For this review, use the dimensioned drawing (mm, ordinates from the lowest corner) and the shaded views. Round coordinates to 2 decimals unless told otherwise and drop trailing zeros. Write each loop counter-clockwise with the first axis right and the second up, starting at its lowest first coordinate (ties: lowest second). Pieces come first, ordered by that corner, then holes. Notation, with made-up numbers: M 58.25,1.25 L 66.25,1.25 A22 cw 66.25,8.25 Z; hole C 83,64 d7. An arc over 180 degrees is marked long. One line per question, with ' | ' between items.
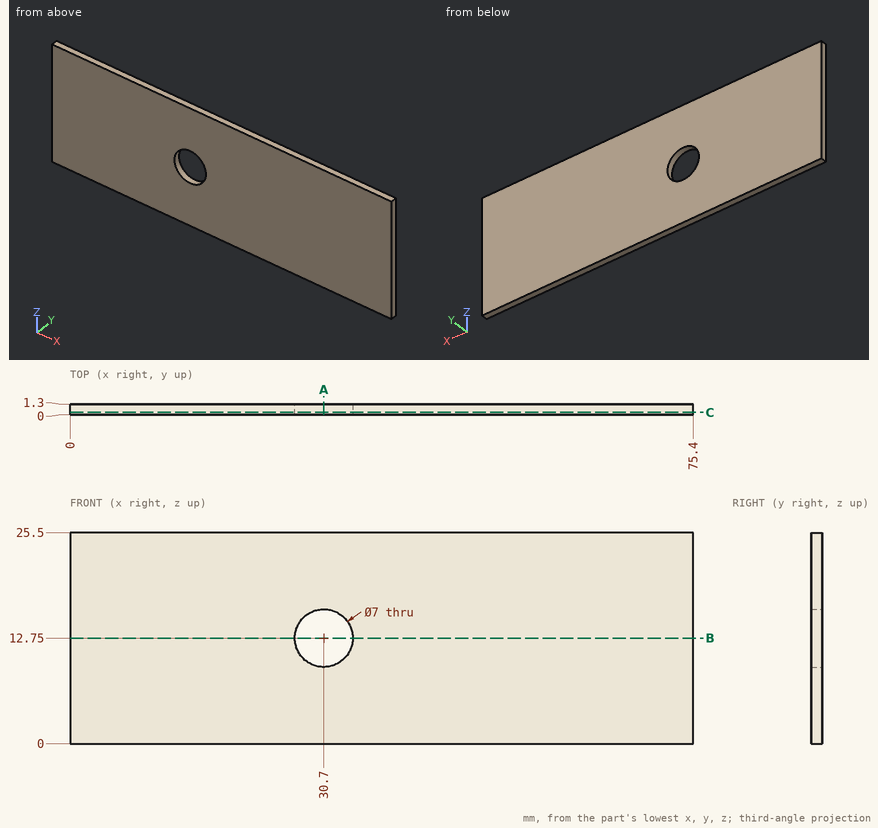
Item 1: Take a section at A-A (x = 30.7). Write out the cut boundary in (y, z).
Results:
outline: M 0,0 L 1.3,0 L 1.3,9.25 L 0,9.25 Z; M 0,16.25 L 1.3,16.25 L 1.3,25.5 L 0,25.5 Z
Item 2: Take a section at B-B (z = 12.75). Write out the cut boundary in (x, y).
Results:
outline: M 0,0 L 27.2,0 L 27.2,1.3 L 0,1.3 Z; M 34.2,0 L 75.4,0 L 75.4,1.3 L 34.2,1.3 Z
Item 3: Take a section at C-C (y = 0.3). Write out the cut boundary in (x, z).
Results:
outline: M 0,0 L 75.4,0 L 75.4,25.5 L 0,25.5 Z; hole C 30.7,12.75 d7
Item 4: To check wall thickness, follow line 1 along Z through (x, y) = (30.7, 0.7); line 2 along X through (y, z) = (0.75, 12.75); line 3 along X through (y, z) = (1.2, 15.5). State the ranges of each line that lie inside material, in increasing order. Write a range as from..to.
Results:
line 1: 0..9.25, 16.25..25.5 | line 2: 0..27.2, 34.2..75.4 | line 3: 0..28.53, 32.87..75.4
Item 5: Insertion check: pin 1 Ø11 at (x, z) = (30.7, 12.75) entering from +Y. The pin has a flat end and moves straight along its axis. Give the tip position at first contact, or say it passes through.
Results:
pin 1: y = 1.3
